CAD build for the part. Positions are in the model's coordinates, mm. Face numbers are marked on the shaded views. Give positions to 0.01 mm unless a question says otherwise; leave off trailing zeros. Loops run counter-clockwise (first coordinate to the right, second up) from the corner with the lowest first, then second, coordinate; pieces in that order, holes last. Notation, with made-up numbers: M -10.75,-8.5 L 26.25,-8.5 A25 ccw 26.25,4.5 Z; hole C 28,56.5 d8. An arc over 180 degrees is marked long. One line per question, with ' | ' between items.
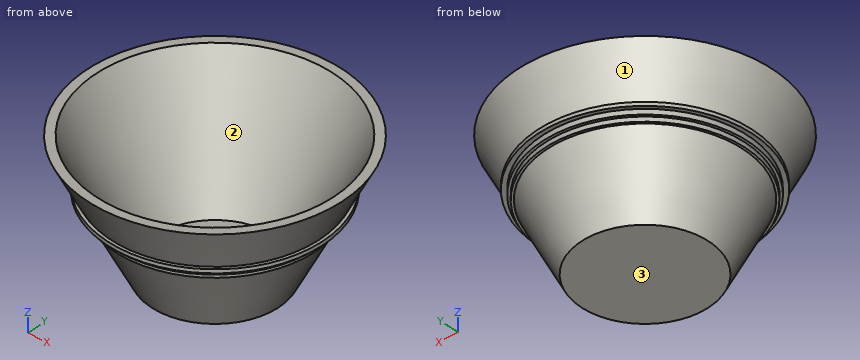
```python
from build123d import *


with BuildPart() as f1:
    # F0 (on Front) → F1 (revolve)
    with BuildSketch(Plane.XZ):
        Polygon((0, 3.0734), (0, 0), (25.4, 0), (39.01757, 27.235139), (39.956536, 29.113071), (40.993106, 31.186212), (41.607701, 32.415403), (50.8, 50.8), (47.363834, 50.8), (23.500534, 3.0734), align=None)
        Polygon((41.607701, 32.415403), (40.993106, 31.186212), (42.863108, 30.934094), (42.863108, 32.415403), align=None)
        Polygon((40.993106, 31.186212), (39.956536, 29.113071), (40.993106, 29.113071), align=None)
        Polygon((39.956536, 29.113071), (39.01757, 27.235139), (39.956536, 27.235139), align=None)
    revolve(axis=Axis((0, 0, 25.4), (0, 0, 1)))


solid = f1.part
```
Item 1: Saw through at D-D on z = 13.5. Give the cut face in (x, y).
Conclusion:
outline: C 0,0 d64.3; hole C 0,0 d57.43
Item 2: Saw through at A-A on y = 0. Give the cut face in (x, z), and give its area (3 significant figures).
Conclusion:
outline: M -50.8,50.8 L -41.61,32.42 L -42.86,32.42 L -42.86,30.93 L -40.99,31.19 L -40.99,29.11 L -39.96,29.11 L -39.96,27.24 L -39.02,27.24 L -25.4,0 L 25.4,0 L 39.02,27.24 L 39.96,27.24 L 39.96,29.11 L 40.99,29.11 L 40.99,31.19 L 42.86,30.93 L 42.86,32.42 L 41.61,32.42 L 50.8,50.8 L 47.36,50.8 L 23.5,3.07 L -23.5,3.07 L -47.36,50.8 Z | area: 497 mm²
Item 3: Drop flat-ended pins along their axis: P1, Ø1.5, axis at y = 23, z = 44.5, coming from the +X side; P2, Ø5, axis at x = 18.5, y = -28, coming from the -Z side; P3, Ø6, axis at x = 0, y = -29.5, coming from the -Z side; P4, Ø10, axis at x = -7, y = 8, coming from the -Z side. Give the stop position or say it passes through.
Conclusion:
P1: x = 42.32 | P2: z = 11.32 | P3: z = 2.2 | P4: z = 0
Item 4: Saw through at C-C on z = 41. Give the cut face in (x, y).
Conclusion:
outline: C 0,0 d91.8; hole C 0,0 d84.93
Item 5: Drill centre lines: line 1 along Y through (x, z) = (-35, 39); line 2 along X through (y, z) = (-5.5, 7.5); line 3 along Z through (x, y) = (-42, -7). Where is each one in solid material? Low to high. Write a range as [from, to].
Conclusion:
line 1: [-28.12, -22.23], [22.23, 28.12] | line 2: [-28.63, -25.12], [25.12, 28.63] | line 3: [30.97, 32.42], [34.36, 41.23]
Item 6: Mould opens along X. For the marked faces 1, 2 and 3 say: pulls with the +X half, pulls with the -X half, needs draft (parallel to the pull), parting line crosses it, or undercut.
Conclusion:
face 1: parting line crosses it | face 2: undercut | face 3: needs draft
